from build123d import *

# Parameters (mm, degrees)
F2_SIZE  = 1
F3_R     = 30
F4_DEPTH = 25
F3_R_2   = 3
F5_DEPTH = 25


with BuildPart() as f1:
    # F0 (on Right) → F1 (revolve)
    with BuildSketch(Plane.YZ):
        Polygon((-20, 7.975), (-20, 6), (10, 6), (10, 8.6), (3.1, 8.6), (3.1, 11.1), (5, 11.1), (5, 21.5), (0, 21.5), (0, 7.175), (-17.5, 7.175), (-17.5, 7.975), align=None)
    revolve(axis=Axis((0, -4.153569, 0), (0, 1, 0)))

    # F2
    f2_edges = [f1.edges().sort_by_distance(p)[0] for p in [
        (0, -20, -7.975),
    ]]
    chamfer(f2_edges, length=F2_SIZE)

    # F3 (on face) → F4 (cut)
    with BuildSketch(Plane.XZ):
        Circle(F3_R)
        with BuildLine():
            ThreePointArc((-17.6, -5.957348), (-21.5, 0), (-17.6, 5.957348))
            Line((-17.6, 5.957348), (-5, 11.456439))
            ThreePointArc((-5, 11.456439), (0, 12.5), (5, 11.456439))
            Line((5, 11.456439), (17.6, 5.957348))
            ThreePointArc((17.6, 5.957348), (21.5, 0), (17.6, -5.957348))
            Line((17.6, -5.957348), (5, -11.456439))
            ThreePointArc((5, -11.456439), (0, -12.5), (-5, -11.456439))
            Line((-5, -11.456439), (-17.6, -5.957348))
        make_face(mode=Mode.SUBTRACT)
    extrude(amount=-F4_DEPTH, mode=Mode.SUBTRACT)

    # F3 (on face) → F5 (cut)
    with BuildSketch(Plane.XZ):
        with Locations((15, 0)):
            Circle(F3_R_2)
        with Locations((-15, 0)):
            Circle(F3_R_2)
    extrude(amount=-F5_DEPTH, mode=Mode.SUBTRACT)


solid = f1.part
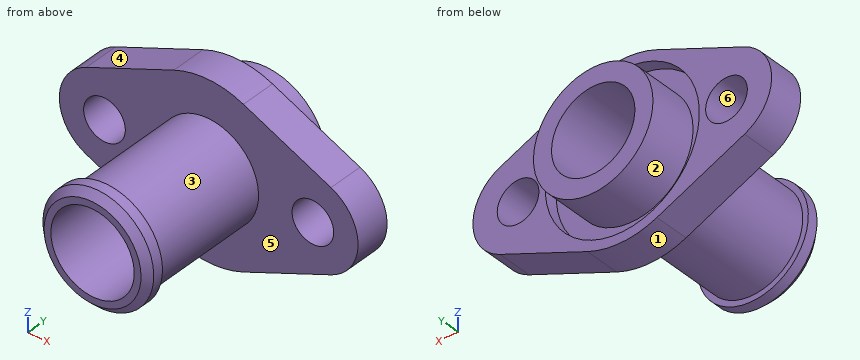
Build history of the part. All positions in model axes, mm. Face numbers are marked on the shaded views. A direction names the side the tool comes from. Coordinates: 2 decimals unless noted, no trailing zeros. Write each loop counter-clockwise with the first axis right and the second up, starting at its lowest first coordinate (ties: lowest second). Pieces come first, ordered by that corner, then holes.
(1) Cut at D-D on z = -9.5. List the corners of the cut face in (x, y), and give its area (3 significant figures).
(2) Cut at C-C on y = -1.5. List the corners of the cut face in (x, z) (3 decimals).
(3) 3-axis set-ups, long thin cutter, end or side, ignore diameter. For the marked faces 1, 2 and 3: which of +Z, -Z, +X, -X, +Y, -Y reach the whole face in a straight line?
(4) Drill centre lines: line 1 (X direction, y = 1.75, z = -0.5); line 2 (X direction, y = 4.75, z = -2.75); line 3 (Y direction, x = 7.5, z = -3). Where is each one in solid material? Low to high.
(5) Cut at A-A on z = 0. State how many separate pieces and enclosed holes the cut face has, and give its area (4 significant figures).
(6) Mould opens along X. For the marked faces 4, 5 and 6 say: pulls with the +X half, pulls with the -X half, needs draft (parallel to the pull), parting line crosses it, or undercut.
(7) Cut at B-B on x = 13. List the corners of the cut face in (y, z).
(8) Pin check, flat tips, straight feed: pin 1 Ø5 at (x, z) = (-12, 5) entering from +Y; pin 2 Ø1 at (x, z) = (6, 9) entering from -Y; pin 3 Ø1.5 at (y, z) = (-8, -1) entering from +X. Stop position of each tip, or through.
Working result:
1. outline: (-9.48, 0) - (9.48, 0) - (9.48, 5) - (5.74, 5) - (5.74, 3.1) - (-5.74, 3.1) - (-5.74, 5) - (-9.48, 5) - close
1. area: 73.0 mm2
2. outline: circle Ø14.35 at (0, 0); hole circle Ø12 at (0, 0)
3. face 1: -Z, +Y, -Y
3. face 2: +Y
3. face 3: none
4. line 1: x = -21.48 to -17.96, -12.04 to -5.98, 5.98 to 12.04, 17.96 to 21.48
4. line 2: x = -20.89 to -16.2, -13.8 to -10.75, -8.15 to -5.33, 5.33 to 8.15, 10.75 to 13.8, 16.2 to 20.89
4. line 3: y = 0 to 10
5. separate pieces: 4
5. enclosed holes: 0
5. area: 161.5 mm2
6. face 4: pulls with the -X half
6. face 5: needs draft
6. face 6: undercut
7. outline: (0, -7.96) - (5, -7.96) - (5, -2.24) - (0, -2.24) - close; (0, 2.24) - (5, 2.24) - (5, 7.96) - (0, 7.96) - close
8. pin 1: stops at y = 5
8. pin 2: stops at y = 0
8. pin 3: stops at x = 7.17
